Read the model definition and answer for the solid it produces. Units are mm, in the model's axes. A direction names the side the tool comes from. Coordinates: 2 decimals unless noted, no trailing zeros. Write each loop counter-clockwise with the first axis right and the second up, starting at its lowest first coordinate (ties: lowest second). Pieces come first, ordered by that corner, then holes.
Item 1: A tool of negligible diameter and unlimited length cuts with its end or side. For faces 1 (the face through (-23, 9, -27.3)), 2 (the face through (-23.021, 8.124, -2.517)), 3 (the face through (-21.5, 7.7, -29.7)), from which of +Z, -Z, +X, -X, +Y, -Y can it reach the whole face along a straight path? Write none if from no direction.
Item 2: Each of these flat-tipped pins is pushed along its axis until it touches: P1, Ø3, axis at x = -18, z = -4, coming from the +Y side; P2, Ø6, axis at y = 13, z = -10, coming from the -X side. Where does it stop, or does it pass through?
Item 3: Determine the mould class of faces 4 (the face through (-23, 15, -30)), 5 (the face through (-23, 9.1, -30.7)), 6 (the face through (-18, 1, -29)) for opening direction Y: released by +Y, released by -Y, zero draft, split by the parting line, or undercut.
Item 4: Section B-B (y = 11.75) is taken. Give the vertices of the cut face in (x, z), then the cut area to 3 significant figures.
Item 5: Section A-A (z = -21.4) is taken. Give the vertices of the cut face in (x, y), then the cut area to 3 significant figures.
Item 6: Section D-D (z = -29.7) is taken. Give the vertices of the cut face in (x, y).
Item 7: Straight lines are drawn through the part: probe 1 along Z at (x, y) = (-5, 0.9); probe 2 along Z at (x, y) = (-23, 10.75); probe 3 along X at (y, z) = (0.5, -20.5). For each, find the intervals that lie inside material, in ascending order.
Item 8: Section C-C (x = -12.6) is taken. Give the vertices of the cut face in (y, z), then the cut area to 3 significant figures.
Autodesk Inventor part; units mm, degrees
ref_plane "YZ Plane" through (0, 0, 0) normal (1, 0, 0) x (0, 1, 0)
ref_plane "XZ Plane" through (0, 0, 0) normal (0, 1, 0) x (-1, 0, 0)
ref_plane "XY Plane" through (0, 0, 0) normal (0, 0, 1) x (1, 0, 0)
sketch "Sketch1" plane through (0, 0, 0) normal (0, 1, 0) x (-1, 0, 0)
  line L0 (0, 0) -> (24.5, 0)
  line L1 (24.5, 0) -> (24.5, -32)
  line L2 (24.5, -32) -> (0, -32)
  line L3 (0, -32) -> (0, 0)
  line L4 (24.5, 0) -> (21.5, 0)
  line L5 (21.5, 0) -> (21.5, -4.7)
  line L6 (21.5, -4.7) -> (24.5, -4.7)
  line L7 (24.5, -4.7) -> (24.5, 0)
  line L8 (24.5, -32) -> (21.5, -32)
  line L9 (21.5, -32) -> (21.5, -27.3)
  line L10 (21.5, -27.3) -> (24.5, -27.3)
  line L11 (24.5, -27.3) -> (24.5, -32)
  line L12 (0, 0) -> (3, 0)
  line L13 (3, 0) -> (3, -32)
  line L14 (3, -32) -> (0, -32)
  line L15 (0, -32) -> (0, 0)
  circle A0 centre (18, -4) radius 1
  circle A1 centre (18, -8) radius 1
  circle A2 centre (18, -24) radius 1
  circle A3 centre (18, -28) radius 1
  circle A4 centre (9, -10.6) radius 1
  circle A5 centre (5, -10.6) radius 1
  circle A6 centre (9, -21.4) radius 1
  circle A7 centre (5, -21.4) radius 1
  circle A8 centre (17, -16) radius 1
  circle A9 centre (12.6, -16) radius 1
  dimension "d0" = 24.5
  dimension "d1" = 32
  dimension "d2" = 3
  dimension "d3" = 4.7
  dimension "d4" = 4.7
  dimension "d5" = 3
  dimension "d6" = 2
  dimension "d7" = 2
  dimension "d8" = 2
  dimension "d9" = 2
  dimension "d10" = 2
  dimension "d11" = 2
  dimension "d12" = 2
  dimension "d13" = 2
  dimension "d14" = 2
  dimension "d15" = 2
  dimension "d16" = 4
  dimension "d17" = 4
  dimension "d18" = 4
  dimension "d19" = 4
  dimension "d20" = 18
  dimension "d21" = 18
  dimension "d22" = 18
  dimension "d23" = 18
  dimension "d24" = 5
  dimension "d25" = 4
  dimension "d26" = 5
  dimension "d27" = 4
  dimension "d28" = 10.6
  dimension "d29" = 10.6
  dimension "d30" = 10.6
  dimension "d31" = 10.6
  dimension "d32" = 16
  dimension "d33" = 16
  dimension "d34" = 4.4
  dimension "d35" = 12.6
  dimension "d36" = 3
extrude "Extrusion1" add sketch "Sketch1" along normal blind 3 contours L0 L5 L6 L1 L10 L9 L2 L13
extrude "Extrusion2" add sketch "Sketch1" along normal blind 15 contours L0 L13 L2 L3 | L0 L1 L6 L5 | L9 L10 L1 L2
sketch "Sketch2" plane through (-24.5, 0, -32) normal (-1, 0, 0) x (0, 0, 1)
  circle A0 centre (29.7, 9.1) radius 1
  circle A1 centre (2.3, 9.1) radius 1
  line L0 (27.3, 15) -> (32, 15)
  line L1 (0, 15) -> (4.7, 15)
  line L2 (32, 0) -> (32, 15)
  line L3 (0, 0) -> (0, 15)
  dimension "d41" = 2
  dimension "d42" = 2
  dimension "d43" = 5.9
  dimension "d44" = 5.9
  dimension "d45" = 2.3
  dimension "d46" = 2.3
extrude "Extrusion3" cut sketch "Sketch2" against normal blind 3
sketch "Sketch3" plane through (0, 0, 0) normal (1, 0, 0) x (0, 0, -1)
  circle A0 centre (10.6, 9) radius 1
  circle A1 centre (21.4, 9) radius 1
  line L0 (0, 15) -> (32, 15)
  line L1 (32, 0) -> (32, 15)
  line L2 (0, 0) -> (0, 15)
  circle A2 centre (16, 9) radius 1
  dimension "d51" = 2
  dimension "d52" = 2
  dimension "d53" = 6
  dimension "d54" = 10.6
  dimension "d55" = 6
  dimension "d56" = 10.6
  dimension "d60" = 2
  dimension "d61" = 6
  dimension "d62" = 16
extrude "Extrusion4" cut sketch "Sketch3" against normal blind 3 contours A0 | A1
fillet "Fillet3" radius 0.5 36 edges at (-24.5, 9, -4.7) (-24.5, 7.5, 0) (-24.5, 15, -2.35) (-24.5, 3, -16) (-24.5, 0, -16) (-24.5, 9, -27.3) (-24.5, 15, -29.65) (-24.5, 7.5, -32) (-12.25, 0, -32) (-12.25, 3, 0) (-23, 3, -4.7) (-23, 15, -4.7) (-23, 15, 0) (-23, 15, -27.3) (-23, 15, -32) (-23, 3, -27.3) (-12.25, 0, 0) (-21.5, 9, 0) (-21.5, 15, -2.35) (-21.5, 9, -27.3) (-21.5, 15, -29.65) (-21.5, 9, -32) (-21.5, 9, -4.7) (-21.5, 3, -2.35) (-21.5, 3, -29.65) (-12.25, 3, -32) (-3, 3, -16) (0, 0, -16) (-3, 9, -32) (0, 7.5, -32) (-1.5, 15, -32) (-3, 15, -16) (0, 15, -16) (-1.5, 15, 0) (-3, 9, 0) (0, 7.5, 0)
extrude "Extrusion5" cut sketch "Sketch3" against normal blind 3 contours A2
properties part number "holder"
Established:
1. face 1: -X, +Y
1. face 2: -X
1. face 3: +Z, -Z, +Y
2. P1: stops at y = 3
2. P2: stops at x = -3
3. face 4: released by +Y
3. face 5: undercut
3. face 6: zero draft
4. outline: (-24.5, -31.5) arc R0.5 ccw to (-24, -32) - (-22, -32) arc R0.5 ccw to (-21.5, -31.5) - (-21.5, -27.8) arc R0.5 ccw to (-22, -27.3) - (-24, -27.3) arc R0.5 ccw to (-24.5, -27.8) - close; (-24.5, -4.2) arc R0.5 ccw to (-24, -4.7) - (-22, -4.7) arc R0.5 ccw to (-21.5, -4.2) - (-21.5, -0.5) arc R0.5 ccw to (-22, 0) - (-24, 0) arc R0.5 ccw to (-24.5, -0.5) - close; (-3, -31.5) arc R0.5 ccw to (-2.5, -32) - (-0.5, -32) arc R0.5 ccw to (0, -31.5) - (0, -0.5) arc R0.5 ccw to (-0.5, 0) - (-2.5, 0) arc R0.5 ccw to (-3, -0.5) - close
4. area: 124 mm2
5. outline: (-24.5, 0.5) arc R0.5 ccw to (-24, 0) - (-10, 0) - (-10, 3) - (-24, 3) arc R0.5 ccw to (-24.5, 2.5) - close; (-8, 0) - (-6, 0) - (-6, 3) - (-8, 3) - close; (-4, 0) - (-0.5, 0) arc R0.5 ccw to (0, 0.5) - (0, 8) - (-3, 8) - (-3, 3.5) arc R0.5 cw to (-3.5, 3) - (-4, 3) - close; (-3, 10) - (0, 10) - (0, 14.5) arc R0.5 ccw to (-0.5, 15) - (-2.5, 15) arc R0.5 ccw to (-3, 14.5) - close
5. area: 91.3 mm2
6. outline: (-24.5, 0.5) arc R0.5 ccw to (-24, 0) - (-0.5, 0) arc R0.5 ccw to (0, 0.5) - (0, 14.5) arc R0.5 ccw to (-0.5, 15) - (-2.5, 15) arc R0.5 ccw to (-3, 14.5) - (-3, 3.5) arc R0.5 cw to (-3.5, 3) - (-21, 3) arc R0.5 cw to (-21.5, 3.5) - (-21.5, 8.1) - (-24.5, 8.1) - close; (-24.5, 10.1) - (-21.5, 10.1) - (-21.5, 14.5) arc R0.5 ccw to (-22, 15) - (-24, 15) arc R0.5 ccw to (-24.5, 14.5) - close
7. probe 1: z = -32 to -22.4, -20.4 to -11.6, -9.6 to 0
7. probe 2: z = -32 to -27.3, -4.7 to 0
7. probe 3: x = -24.5 to -9.44, -8.56 to -5.44, -4.56 to 0
8. outline: (0, -31.5) arc R0.5 ccw to (0.5, -32) - (2.5, -32) arc R0.5 ccw to (3, -31.5) - (3, -17) - (0, -17) - close; (0, -15) - (3, -15) - (3, -0.5) arc R0.5 ccw to (2.5, 0) - (0.5, 0) arc R0.5 ccw to (0, -0.5) - close
8. area: 89.8 mm2
